```python
from build123d import *

# Parameters (mm, degrees)
SKETCH1_R           = 1.6
BOSS_EXTRUDE1_DEPTH = 6
SKETCH2_W           = 2.5
SKETCH2_H           = 42
SKETCH2_H_2         = 8
SKETCH2_H_3         = 6
SKETCH2_W_2         = 13
SKETCH2_W_3         = 2
SKETCH2_W_4         = 3
SKETCH2_H_4         = 10
BOSS_EXTRUDE2_DEPTH = 7.5
FILLET3_R           = 4
FILLET4_R           = 4


with BuildPart() as part:
    # Sketch1 → Boss-Extrude1 (new body)
    with BuildSketch(Plane(origin=(0, 0, 0), x_dir=(1, 0, 0), z_dir=(0, 1, 0))):
        with BuildLine():
            Line((-4, -16.5), (0, -16.5))
            ThreePointArc((0, -16.5), (2.828427125, -15.328427125), (4, -12.5))
            Line((4, -12.5), (4, 12.5))
            ThreePointArc((4, 12.5), (2.828427125, 15.328427125), (0, 16.5))
            Line((0, 16.5), (-4, 16.5))
            Line((-4, 16.5), (-4, -16.5))
        make_face()
        with Locations(Location((0, 12.5, 0), (0, 0, 270))):
            Circle(SKETCH1_R, mode=Mode.SUBTRACT)
        with Locations(Location((0, -12.5, 0), (0, 0, 270))):
            Circle(SKETCH1_R, mode=Mode.SUBTRACT)
        with Locations(Location((0, 0, 0), (0, 0, 270))):
            Circle(SKETCH1_R, mode=Mode.SUBTRACT)
    extrude(amount=BOSS_EXTRUDE1_DEPTH)

    # Sketch2 → Boss-Extrude2 (add)
    with BuildSketch(Plane.ZY.offset(4)):
        with BuildLine():
            Line((14.5, 49.877005851), (14.5, 99.877005851))
            ThreePointArc((14.5, 99.877005851), (13.81662479, 97.640937873), (12, 96.168906607))
            Line((12, 96.168906607), (12, 53.585105094))
            ThreePointArc((12, 53.585105094), (13.81662479, 52.113073828), (14.5, 49.877005851))
        make_face()
        with Locations((7.75, 74.877005851)):
            Rectangle(SKETCH2_W, SKETCH2_H)
        with BuildLine():
            ThreePointArc((14.5, 99.877005851), (13.328427125, 102.705432976), (10.5, 103.877005851))
            ThreePointArc((10.5, 103.877005851), (7.671572875, 102.705432976), (6.5, 99.877005851))
            Line((6.5, 99.877005851), (6.5, 95.877005851))
            Line((6.5, 95.877005851), (9, 95.877005851))
            Line((9, 95.877005851), (9, 99.877005851))
            ThreePointArc((9, 99.877005851), (10.5, 101.377005851), (12, 99.877005851))
            Line((12, 99.877005851), (12, 96.168906607))
            ThreePointArc((12, 96.168906607), (13.81662479, 97.640937873), (14.5, 99.877005851))
        make_face()
        with BuildLine():
            Line((10.5, 103.877005851), (-10.5, 103.877005851))
            ThreePointArc((-10.5, 103.877005851), (-7.671572875, 102.705432976), (-6.5, 99.877005851))
            Line((-6.5, 99.877005851), (-6.5, 95.877005851))
            Line((-6.5, 95.877005851), (6.5, 95.877005851))
            Line((6.5, 95.877005851), (6.5, 99.877005851))
            ThreePointArc((6.5, 99.877005851), (7.671572875, 102.705432976), (10.5, 103.877005851))
        make_face()
        with BuildLine():
            ThreePointArc((-10.5, 103.877005851), (-13.328427125, 102.705432976), (-14.5, 99.877005851))
            ThreePointArc((-14.5, 99.877005851), (-13.81662479, 97.640937873), (-12, 96.168906607))
            Line((-12, 96.168906607), (-12, 99.877005851))
            ThreePointArc((-12, 99.877005851), (-10.5, 101.377005851), (-9, 99.877005851))
            Line((-9, 99.877005851), (-9, 95.877005851))
            Line((-9, 95.877005851), (-6.5, 95.877005851))
            Line((-6.5, 95.877005851), (-6.5, 99.877005851))
            ThreePointArc((-6.5, 99.877005851), (-7.671572875, 102.705432976), (-10.5, 103.877005851))
        make_face()
        with BuildLine():
            Line((-14.5, 99.877005851), (-14.5, 49.877005807))
            ThreePointArc((-14.5, 49.877005807), (-13.816624803, 52.11307381), (-12, 53.585105094))
            Line((-12, 53.585105094), (-12, 96.168906607))
            ThreePointArc((-12, 96.168906607), (-13.81662479, 97.640937873), (-14.5, 99.877005851))
        make_face()
        with Locations((-7.75, 74.877005851)):
            Rectangle(SKETCH2_W, SKETCH2_H)
        with Locations((7.75, 49.877005851)):
            Rectangle(SKETCH2_W, SKETCH2_H_2)
        with BuildLine():
            ThreePointArc((12, 46.168906607), (13.81662479, 47.640937873), (14.5, 49.877005851))
            ThreePointArc((14.5, 49.877005851), (13.81662479, 52.113073828), (12, 53.585105094))
            Line((12, 53.585105094), (12, 46.168906607))
        make_face()
        with Locations((-7.75, 49.877005851)):
            Rectangle(SKETCH2_W, SKETCH2_H_2)
        with BuildLine():
            ThreePointArc((-12, 53.585105094), (-13.816624803, 52.11307381), (-14.5, 49.877005807))
            ThreePointArc((-14.5, 49.877005807), (-13.816624778, 47.640937855), (-12, 46.168906607))
            Line((-12, 46.168906607), (-12, 53.585105094))
        make_face()
        with BuildLine():
            Line((-14.5, 49.877005807), (-14.5, 6))
            Line((-14.5, 6), (-12, 6))
            Line((-12, 6), (-12, 16))
            Line((-12, 16), (-12, 46.168906607))
            ThreePointArc((-12, 46.168906607), (-13.816624778, 47.640937855), (-14.5, 49.877005807))
        make_face()
        with BuildLine():
            Line((12, 16), (12, 6))
            Line((12, 6), (14.5, 6))
            Line((14.5, 6), (14.5, 49.877005851))
            ThreePointArc((14.5, 49.877005851), (13.81662479, 47.640937873), (12, 46.168906607))
            Line((12, 46.168906607), (12, 16))
        make_face()
        Polygon((6.5, 45.877005851), (6.5, 6), (9, 6), (9, 16), (9, 45.877005851), align=None)
        with Locations((13.25, 3)):
            Rectangle(SKETCH2_W, SKETCH2_H_3)
        with Locations((7.75, 3)):
            Rectangle(SKETCH2_W, SKETCH2_H_3)
        with Locations((-7.75, 3)):
            Rectangle(SKETCH2_W, SKETCH2_H_3)
        with Locations((-13.25, 3)):
            Rectangle(SKETCH2_W, SKETCH2_H_3)
        Polygon((-9, 6), (-6.5, 6), (-6.5, 45.877005851), (-9, 45.877005851), (-9, 16), align=None)
        with Locations((0, 3)):
            Rectangle(SKETCH2_W_2, SKETCH2_H_3)
        with Locations((-15.5, 3)):
            Rectangle(SKETCH2_W_3, SKETCH2_H_3)
        with Locations((-10.5, 3)):
            Rectangle(SKETCH2_W_4, SKETCH2_H_3)
        with Locations((15.5, 3)):
            Rectangle(SKETCH2_W_3, SKETCH2_H_3)
        with Locations((10.5, 3)):
            Rectangle(SKETCH2_W_4, SKETCH2_H_3)
        with Locations((0, 49.877005851)):
            Rectangle(SKETCH2_W_2, SKETCH2_H_2)
        with Locations((-10.5, 11)):
            Rectangle(SKETCH2_W_4, SKETCH2_H_4)
        with Locations((10.5, 11)):
            Rectangle(SKETCH2_W_4, SKETCH2_H_4)
    extrude(amount=BOSS_EXTRUDE2_DEPTH)

    # Fillet3
    # the kernel refuses this fillet: 4 mm, written as the material it adds along each edge
    with BuildSketch(Plane(origin=(-4, 6, 6.5), x_dir=(0, 0, -1), z_dir=(-1, 0, 0))) as fillet3_piece_1:
        with BuildLine():
            CenterArc((FILLET3_R, -FILLET3_R), FILLET3_R, 90, 90)
            Line((0, -FILLET3_R), (-FILLET3_R * 0.02, -FILLET3_R))
            Line((-FILLET3_R * 0.02, -FILLET3_R), (-FILLET3_R * 0.02, FILLET3_R * 0.02))
            Line((-FILLET3_R * 0.02, FILLET3_R * 0.02), (FILLET3_R, FILLET3_R * 0.02))
            Line((FILLET3_R, FILLET3_R * 0.02), (FILLET3_R, 0))
        make_face()
    extrude(amount=7.5)
    with BuildSketch(Plane(origin=(-4, 6, -14.5), x_dir=(0, 0, -1), z_dir=(-1, 0, 0))) as fillet3_piece_2:
        with BuildLine():
            CenterArc((4, -3.464101615), FILLET3_R, 120, 60)
            Line((0, -3.464101615), (-0.08, -3.464101615))
            Line((-0.08, -3.464101615), (-0.08, 0))
            Line((-0.08, 0), (0, 0.08))
            ThreePointArc((0, 0.08), (1, 0.08), (1.96, 0.069282032))
            Line((1.96, 0.069282032), (2, 0))
        make_face()
    extrude(amount=7.5)
    with BuildSketch(Plane(origin=(-4, 6, 14.5), x_dir=(0, 0, 1), z_dir=(-1, 0, 0))) as fillet3_piece_3:
        with BuildLine():
            CenterArc((4, 3.464101615), FILLET3_R, 180, 60)
            Line((0, 3.464101615), (-0.08, 3.464101615))
            Line((-0.08, 3.464101615), (-0.08, 0))
            Line((-0.08, 0), (0, -0.08))
            ThreePointArc((0, -0.08), (1, -0.08), (1.96, -0.069282032))
            Line((1.96, -0.069282032), (2, 0))
        make_face()
    extrude(amount=7.5)
    with BuildSketch(Plane(origin=(-4, 6, -6.5), x_dir=(0, 0, 1), z_dir=(-1, 0, 0))) as fillet3_piece_4:
        with BuildLine():
            CenterArc((FILLET3_R, FILLET3_R), FILLET3_R, 180, 90)
            Line((0, FILLET3_R), (-FILLET3_R * 0.02, FILLET3_R))
            Line((-FILLET3_R * 0.02, FILLET3_R), (-FILLET3_R * 0.02, -FILLET3_R * 0.02))
            Line((-FILLET3_R * 0.02, -FILLET3_R * 0.02), (FILLET3_R, -FILLET3_R * 0.02))
            Line((FILLET3_R, -FILLET3_R * 0.02), (FILLET3_R, 0))
        make_face()
    extrude(amount=7.5)

    # Fillet4
    fillet4_edges = [part.edges().sort_by_distance(p)[0] for p in [
        (-7.75, 45.877005851, -6.5),
        (-7.75, 45.877005851, 6.5),
        (-7.75, 95.877005851, -6.5),
        (-7.75, 95.877005851, 6.5),
        (-7.75, 53.877005851, 6.5),
        (-7.75, 53.877005851, -6.5),
    ]]
    fillet(fillet4_edges, radius=FILLET4_R)


solid = part.part
```
Geometry: final body of the model. Coordinates: model frame, mm. A direction names the side the tool comes from. Give positions to 0.01 mm unless a question says otherwise; leave off trailing zeros. Loops run counter-clockwise (first coordinate to the right, second up) from the corner with the lowest first, then second, coordinate; pieces in that order, holes last. Notation, with made-up numbers: (-3, 74) -> (13, 74) arc R24 cw to (13, 92) -> close; hole circle Ø9 at (9, 86.5). An arc over 180 degrees is marked (long way). Use one line per item in the form item = value.
Item 1: Section query D-D on x = -2.5. Output: boundary loops of the cut face in (y, z).
A:
outline = (0, -16.5) -> (6, -16.5) -> (6, 16.5) -> (0, 16.5) -> close
Item 2: Draft query along Z for faces 1 (the face through (-7.7, 7.44, -15.05)), 2 (the face through (2.797, 2.958, 15.359)), 3 (the face through (-7.698, 101.377, -10.533)). Return one class per face: pulls with the +Z half, pulls with the -Z half, needs draft (parallel to the pull), parting line crosses it, or undercut.
A:
face_1 = pulls with the -Z half
face_2 = pulls with the +Z half
face_3 = undercut
Item 3: Line query: probe 1 along Y at (x, z) = (-6.25, 2); probe 2 along X at (y, z) = (1.2, -12.5); probe 3 along Z at (x, y) = (-9, 91). Output: solid intervals per line, ascending.
A:
probe_1 = 0 to 6, 45.88 to 53.88, 95.88 to 103.88
probe_2 = -11.5 to -1.6, 1.6 to 4
probe_3 = -14.5 to -12, -9 to -6.5, 6.5 to 9, 12 to 14.5
Item 4: Access query for faces 4 (the face through (-7.698, 101.377, 10.467)), 5 (the face through (-8, 55, -14.5)), 6 (the face through (0.07, 2.96, -14.1)), 7 (the face through (4, 3, 0)), 8 (the face through (-8, 54, 14.5)). Directions: +Z, -Z, +X, -X, +Y, -Y. A direction counts if a zero-diameter tool reaches every point of the face in a straight line with its end or side. Return the directions, or none.
A:
face_4 = +X, -X
face_5 = -Z, +X, -X, +Y
face_6 = +Y, -Y
face_7 = +Z, -Z, +X, +Y, -Y
face_8 = +Z, +X, -X, +Y
Item 5: Section query A-A on y = 17.5. Output: boundary loops of the cut face in (x, z), and give its area (3 significant figures).
A:
outline = (-11.5, -14.5) -> (-4, -14.5) -> (-4, -12) -> (-11.5, -12) -> close; (-11.5, -9) -> (-4, -9) -> (-4, -6.5) -> (-11.5, -6.5) -> close; (-11.5, 6.5) -> (-4, 6.5) -> (-4, 9) -> (-11.5, 9) -> close; (-11.5, 12) -> (-4, 12) -> (-4, 14.5) -> (-11.5, 14.5) -> close
area = 75.0 mm^2
Item 6: Pin query (flat end, axial travel): P1, Ø4, axis at x = -6, y = 29.5, coming from the +Z side; P2, Ø4, axis at x = -8, y = 30.5, coming from the -Z side; P3, Ø10, axis at y = 60, z = 8, coming from the +X side. Return the tip coordinate at first contact, or that it passes through.
A:
P1 = 14.5
P2 = -14.5
P3 = -4
Item 7: Section query C-C on z = 0. Output: boundary loops of the cut face in (x, y), and give its area (3 significant figures).
A:
outline = (-11.5, 0) -> (-1.6, 0) -> (-1.6, 6) -> (-11.5, 6) -> close; (-11.5, 45.88) -> (-4, 45.88) -> (-4, 53.88) -> (-11.5, 53.88) -> close; (-11.5, 95.88) -> (-4, 95.88) -> (-4, 103.88) -> (-11.5, 103.88) -> close; (1.6, 0) -> (4, 0) -> (4, 6) -> (1.6, 6) -> close
area = 194 mm^2
Item 8: Section query B-B on x = -9. Give the number of separate pieces and of enclosed holes in the cut face, and give its area (3 significant figures).
A:
separate_pieces = 1
enclosed_holes = 4
area = 1,490 mm^2
